Check sheet for the modelled part. Datum: model origin and axes. Units: mm. Round coordinates to 2 decimals unless told otherwise and drop trailing zeros. Write each loop counter-clockwise with the first axis right and the second up, starting at its lowest first coordinate (ties: lowest second). Pieces come first, ordered by that corner, then holes. Notation, with made-up numbers: M -35,71 L 18,71 A23 cw 18,97 Z; hole C 3,30.25 d11. An arc over 180 degrees is marked long. Answer in a Markdown table with one row per item.
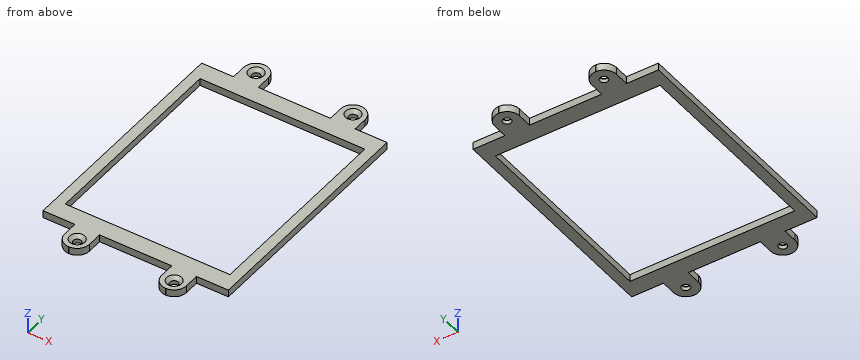
```python
from build123d import *

# Parameters (mm, degrees)
SKETCH045_R      = 1.7
EXTRUDE003_DEPTH = 4
EXTRUDE004_DEPTH = 3
CHAMFER001_SIZE  = 1.4


with BuildPart() as extrude003:
    # Sketch045 → Extrude003 (new body)
    with BuildSketch(Plane.XY):
        with Locations((10.555, 54.404)):
            Circle(SKETCH045_R)
        with Locations((50.555, 54.404)):
            Circle(SKETCH045_R)
        with Locations((10.555, -54.404)):
            Circle(SKETCH045_R)
        with Locations((50.555, -54.404)):
            Circle(SKETCH045_R)
    extrude(amount=EXTRUDE003_DEPTH)


with BuildPart() as pcbholder:
    # Sketch044 → Extrude004 (new body)
    with BuildSketch(Plane.XY):
        with BuildLine():
            Line((68.759, -48.254), (68.759, 48.254))
            Line((55.605, 48.254), (68.759, 48.254))
            Line((55.605, 48.254), (55.605, 54.404))
            ThreePointArc((55.605, 54.404), (54.125889, 57.974889), (50.555, 59.454))
            Line((50.555, 59.454), (50.455, 59.454))
            ThreePointArc((50.455, 59.454), (46.884111, 57.974889), (45.405, 54.404))
            Line((45.405, 54.404), (45.405, 48.254))
            Line((15.605, 48.254), (45.405, 48.254))
            Line((15.605, 48.254), (15.605, 54.404))
            ThreePointArc((15.605, 54.404), (14.125889, 57.974889), (10.555, 59.454))
            Line((10.555, 59.454), (10.455, 59.454))
            ThreePointArc((10.455, 59.454), (6.884111, 57.974889), (5.405, 54.404))
            Line((5.405, 54.404), (5.405, 48.254))
            Line((-7.749, 48.254), (5.405, 48.254))
            Line((-7.749, 48.254), (-7.749, 0))
            Line((-7.749, 0), (-7.749, -48.254))
            Line((-7.749, -48.254), (5.405, -48.254))
            Line((5.405, -48.254), (5.405, -54.404))
            ThreePointArc((5.405, -54.404), (6.884111, -57.974889), (10.455, -59.454))
            Line((10.455, -59.454), (10.555, -59.454))
            ThreePointArc((10.555, -59.454), (14.125889, -57.974889), (15.605, -54.404))
            Line((15.605, -54.404), (15.605, -48.254))
            Line((15.605, -48.254), (45.405, -48.254))
            Line((45.405, -48.254), (45.405, -54.404))
            ThreePointArc((45.405, -54.404), (46.884111, -57.974889), (50.455, -59.454))
            Line((50.455, -59.454), (50.555, -59.454))
            ThreePointArc((50.555, -59.454), (54.125889, -57.974889), (55.605, -54.404))
            Line((55.605, -54.404), (55.605, -48.254))
            Line((55.605, -48.254), (68.759, -48.254))
        make_face()
        Polygon((-3.495, 41), (-3.495, -41), (64.505, -41), (64.505, 41), (30.505, 41), align=None, mode=Mode.SUBTRACT)
    extrude(amount=EXTRUDE004_DEPTH)

    # Cut: cut Extrude003
    add(extrude003.part, mode=Mode.SUBTRACT)

    # Chamfer001
    chamfer001_edges = [pcbholder.edges().sort_by_distance(p)[0] for p in [
        (8.855, 54.404, 3),
        (48.855, 54.404, 3),
        (8.855, -54.404, 3),
        (48.855, -54.404, 3),
    ]]
    chamfer(chamfer001_edges, length=CHAMFER001_SIZE)


with BuildPart() as pcbholder_1:
    # Body004 placement: moved
    add(pcbholder.part.moved(Location((0, 0, -44.4))))


solid = pcbholder_1.part
```
1. Section check C-C, the plane z = -43.25. Count the separate pieces of the cut face and the enclosed holes in it, and give its area (3 significant figures).
Found:
| item | result |
|---|---|
| separate pieces | 1 |
| enclosed holes | 5 |
| area | 2,180 mm2 |
2. Go/stop test with flat-tipped pins: pin 1 (2.5 mm diameter, centred on x = 50.555, y = -54.404, fed in from -Z); pin 2 (0.9 mm diameter, centred on y = 52.5, z = -43.5, fed in from -X) (3 decimals); pin 3 (0.9 mm diameter, centred on x = 1, z = -43, fed in from -Y); pin 4 (4 mm diameter, centred on x = 10.555, y = 54.404, fed in from +Z). Record where each tip stops, or that it passes through.
Found:
| item | result |
|---|---|
| pin 1 | passes through |
| pin 2 | stops at x = 5.405 |
| pin 3 | stops at y = -48.25 |
| pin 4 | stops at z = -42.5 |
3. Section check B-B, the plane y = -3.5. Record the cut outline in (x, z) (3 decimals), and give its area (3 significant figures).
Found:
| item | result |
|---|---|
| outline | M -7.749,-44.4 L -3.495,-44.4 L -3.495,-41.4 L -7.749,-41.4 Z; M 64.505,-44.4 L 68.759,-44.4 L 68.759,-41.4 L 64.505,-41.4 Z |
| area | 25.5 mm2 |
4. Section check A-A, the plane x = 25. Record the cut outline in (y, z).
Found:
| item | result |
|---|---|
| outline | M -48.25,-44.4 L -41,-44.4 L -41,-41.4 L -48.25,-41.4 Z; M 41,-44.4 L 48.25,-44.4 L 48.25,-41.4 L 41,-41.4 Z |
5. Scan lines: L1, parallel to Y at x = 10.5, z = -44.1; L2, parallel to Y at x = 60.5, z = -43.65; L3, parallel to X at y = -9, z = -42.2 (3 decimals). Record each from-to range of solid material in increasing order.
Found:
| item | result |
|---|---|
| L1 | y = -59.45 to -56.1, -52.7 to -41, 41 to 52.7, 56.1 to 59.45 |
| L2 | y = -48.25 to -41, 41 to 48.25 |
| L3 | x = -7.749 to -3.495, 64.505 to 68.759 |
